Here's how the part is built. I have some questions about the finished solid (model axes, mm). A direction names the side the tool comes from. Give positions to 0.01 mm unless a question says otherwise; leave off trailing zeros. Order: outer loops, then holes, each group sorted by start corner. A loop starts at its lowest first (then second) coordinate and runs counter-clockwise, first axis right, second up. Notation, with made-up numbers: (11, 69) - (61, 69) arc R19 ccw to (61, 93) - close; hole circle Ø8 at (-33, -27). An arc over 180 degrees is marked (long way). One line per question, with ' | ' between items.
from build123d import *
from build123d.topology import SkipClean

# Parameters (mm, degrees)
BOSS_EXTRUDE1_DEPTH   = 3.81
BODY_MOVE_COPY2_ANGLE = 180
BOSS_EXTRUDE2_START   = -25.4
SKETCH2_R             = 9.5
BOSS_EXTRUDE2_DEPTH   = 146.05
LPATTERN1_COUNT       = 3
LPATTERN1_PITCH       = 146.05
BODY_MOVE_COPY3_ANGLE = 120
BODY_MOVE_COPY4_ANGLE = 120
BOSS_EXTRUDE3_START   = 27.94
SKETCH3_R             = 9.5
BOSS_EXTRUDE3_DEPTH   = 27.94
SKETCH5_R             = 9.5
BOSS_EXTRUDE4_DEPTH   = 25.4


with BuildPart() as part:
    # Sketch1 → Boss-Extrude1 (new, symmetric)
    with BuildSketch(Plane.XY):
        with BuildLine():
            Line((-5.499261314, 15.875), (-10.998522628, 6.35))
            ThreePointArc((-10.998522628, 6.35), (0, -12.7), (10.998522628, 6.35))
            Line((10.998522628, 6.35), (5.499261314, 15.875))
            ThreePointArc((5.499261314, 15.875), (0, 19.05), (-5.499261314, 15.875))
        make_face()
    extrude(amount=BOSS_EXTRUDE1_DEPTH, both=True)


with BuildPart() as body_2:
    # Body-Move_Copy1: copy of part
    add(part.part.moved(Location((0, 0, 60.96))))


with BuildPart() as part_1:
    # Body-Move_Copy2: moved
    add(part.part.rotate(Axis((0, 0, 0), (0, 0, 1)), BODY_MOVE_COPY2_ANGLE))


    add(body_2.part)  # Boss-Extrude2 merges body 2
    # Sketch2 → Boss-Extrude2 (add)
    with BuildSketch(Plane.XY.offset(BOSS_EXTRUDE2_START)):
        Circle(SKETCH2_R)
    extrude(amount=BOSS_EXTRUDE2_DEPTH)


with BuildPart() as lpattern1_1:
    # LPattern1: pattern copy
    add(part_1.part.moved(Location(Vector(0, 0, 1) * (1 * LPATTERN1_PITCH))))


with BuildPart() as lpattern1_2:
    # LPattern1: pattern copy
    add(part_1.part.moved(Location(Vector(0, 0, 1) * (2 * LPATTERN1_PITCH))))


with BuildPart() as lpattern1_1_1:
    # Body-Move_Copy3: moved
    add(lpattern1_1.part.rotate(Axis((0, 0, 0), (0, 0, 1)), BODY_MOVE_COPY3_ANGLE))


with BuildPart() as lpattern1_2_1:
    # Body-Move_Copy4: moved
    add(lpattern1_2.part.rotate(Axis((0, 0, 0), (0, 0, -1)), BODY_MOVE_COPY4_ANGLE))


with BuildPart() as part_2:
    with SkipClean():  # the faces are left unmerged after this step: merging them gives an invalid solid
        add(part_1.part)

        # Sketch3 → Boss-Extrude3 (add)
        with BuildSketch(Plane(origin=(0, 0, -25.4), x_dir=(-1, 0, 0), z_dir=(0, 0, -1)).offset(BOSS_EXTRUDE3_START)):
            with Locations(Location((0, 0, 0), (0, 0, 300))):
                Circle(SKETCH3_R)
        extrude(amount=-BOSS_EXTRUDE3_DEPTH)

    # Combine1: union LPattern1_1, LPattern1_2
    add(lpattern1_1_1.part)
    add(lpattern1_2_1.part)

    # Sketch5 → Boss-Extrude4 (add)
    with SkipClean():  # the faces are left unmerged after this step: merging them gives an invalid solid
        with BuildSketch(Plane.XY.offset(412.75)):
            Circle(SKETCH5_R)
        extrude(amount=BOSS_EXTRUDE4_DEPTH)


solid = part_2.part
1) Thinking about a two-plate mould opening in Z: for faces 1 (the face through (-0.09, -19.05, 0.05)), 2 (the face through (7, -7, 356.87)), 3 (the face through (-7, 7, 288.29)), 4 (the face through (-9.102, -2.72, 249.013)), which applies, +Z half, -Z half, draft (parallel to the pull), parting line (faces both ways), or undercut?
Model answer:
face 1: draft | face 2: +Z half | face 3: undercut | face 4: undercut
2) I want a section at A-A (z = 190). List the corners of the cut face in (x, y) for me.
Model answer:
outline: circle Ø19 at (0, 0)
3) Please list where these lines run through material, in increasing order: L1, parallel to Z at x = -3, y = 11; L2, parallel to Z at x = -8.5, y = -10; L3, parallel to Z at x = -3, y = -16.5.
Model answer:
L1: z = -3.81 to 3.81, 57.15 to 64.77, 142.24 to 149.86, 203.2 to 210.82, 288.29 to 295.91, 349.25 to 356.87 | L2: z = -3.81 to 3.81, 203.2 to 210.82 | L3: z = -3.81 to 3.81
4) On a 3-axis mill with a long thin cutter (end or side, diameter ignored), from which of +Z, -Z, +X, -X, +Y, -Y can I reach the whole of each face in a straight line? I mean faces 5 (the face through (5, -12.7, 353)), 6 (the face through (-13.8, -1.5, 292.2)), 7 (the face through (7, -7, 349.25)), 8 (the face through (6, 12.7, 146)). Say none if no direction works.
Model answer:
face 5: +Z, +X, -X, -Y | face 6: +Z, -X, -Y | face 7: none | face 8: +Z, +X, -X, +Y
5) I'm going to push flat-ended pins straight in: P1, Ø1, axis at x = -5.5, z = 84, coming from the -Y side; P2, Ø4, axis at x = -7.5, z = 206, coming from the -Y side; P3, Ø10, axis at y = -7.5, z = 162, coming from the +X side; P4, Ø1, axis at y = 10.5, z = 151, coming from the +X side. Where does each tip first touch, or does it pass through?
Model answer:
P1: stops at y = -8.08 | P2: stops at y = -12.7 | P3: stops at x = 9.17 | P4: passes through
